The model under review builds one solid part; all positions refer to its coordinate system, in mm. Coordinates: 2 decimals unless noted, no trailing zeros. Loops run counter-clockwise (first coordinate to the right, second up) from the corner with the lowest first, then second, coordinate; pieces in that order, holes last. Notation, with made-up numbers: M -21.75,18 L 12.25,18 A15 cw 12.25,33 Z; hole C 52,16.5 d2. An arc over 180 degrees is marked long. Use CSV: the item, a comma, the result in double quotes. Start each with the question number.
from build123d import *

# Parameters (mm, degrees)
SKETCH_1_R          = 6
EXTRUDE_1_DEPTH     = 3
SKETCH_2_R          = 2.5
SKETCH_2_W          = 12
SKETCH_2_H          = 28
SKETCH_2_W_2        = 10
CUT_EXTRUDE_1_DEPTH = 725.098439741
SKETCH_3_W          = 6.5
SKETCH_3_H          = 275.47
EXTRUDE_2_DEPTH     = 3
SKETCH_4_W          = 602.3
SKETCH_4_H          = 15
EXTRUDE_3_DEPTH     = 3
FILLET_1_R          = 4


with BuildPart() as part:
    # 草图1 → 凸台-拉伸1 (new body)
    with BuildSketch(Plane.XY):
        with BuildLine():
            Line((64.592959067, -287.27493325), (-37.121356584, -436.580350718))
            ThreePointArc((-37.121356584, -436.580350718), (-39.401099826, -438.618784839), (-42.369287668, -439.355197667))
            Line((-42.369287668, -439.355197667), (-87.565404468, -439.355197667))
            ThreePointArc((-87.565404468, -439.355197667), (-90.533592309, -438.618784839), (-92.813335552, -436.580350718))
            Line((-92.813335552, -436.580350718), (-194.527651202, -287.27493325))
            Line((-194.527651202, -287.27493325), (-376.117346068, -287.27493325))
            Line((-376.117346068, -287.27493325), (-376.117346068, -612.39493325))
            ThreePointArc((-376.117346068, -612.39493325), (-374.257474128, -616.885061311), (-369.767346068, -618.74493325))
            Line((-369.767346068, -618.74493325), (239.832653932, -618.74493325))
            ThreePointArc((239.832653932, -618.74493325), (244.322781993, -616.885061311), (246.182653932, -612.39493325))
            Line((246.182653932, -612.39493325), (246.182653932, -287.27493325))
            Line((246.182653932, -287.27493325), (64.592959067, -287.27493325))
        make_face()
        with Locations((-111.371152168, -477.768197584)):
            Circle(SKETCH_1_R, mode=Mode.SUBTRACT)
        with Locations((-18.563539968, -477.768197584)):
            Circle(SKETCH_1_R, mode=Mode.SUBTRACT)
        with Locations((239.832653932, -607.63243325)):
            Circle(SKETCH_1_R, mode=Mode.SUBTRACT)
        with Locations((239.832653932, -594.93243325)):
            Circle(SKETCH_1_R, mode=Mode.SUBTRACT)
        with Locations(Location((-369.767346068, -607.63243325, 0), (0, 0, 180))):
            Circle(SKETCH_1_R, mode=Mode.SUBTRACT)
        with Locations(Location((-369.767346068, -594.93243325, 0), (0, 0, 180))):
            Circle(SKETCH_1_R, mode=Mode.SUBTRACT)
        with BuildLine():
            Line((-120.598278576, -553.999595792), (-117.888346515, -540.449935487))
            Line((-117.888346515, -540.449935487), (-113.593422095, -518.975313388))
            Line((-113.593422095, -518.975313388), (-109.909811627, -500.557261048))
            ThreePointArc((-109.909811627, -500.557261048), (-109.015545442, -498.354731753), (-107.373986867, -496.635390964))
            Line((-107.373986867, -496.635390964), (-68.658208598, -468.981263629))
            ThreePointArc((-68.658208598, -468.981263629), (-64.967346068, -467.798471171), (-61.276483538, -468.981263629))
            Line((-61.276483538, -468.981263629), (-22.560705269, -496.635390964))
            ThreePointArc((-22.560705269, -496.635390964), (-20.919146693, -498.354731753), (-20.024880508, -500.557261048))
            Line((-20.024880508, -500.557261048), (-16.34127004, -518.975313388))
            Line((-16.34127004, -518.975313388), (-12.04634562, -540.449935487))
            Line((-12.04634562, -540.449935487), (-9.336413559, -553.999595792))
            ThreePointArc((-9.336413559, -553.999595792), (-10.652378252, -559.270762801), (-15.56310085, -561.59493325))
            Line((-15.56310085, -561.59493325), (-114.371591285, -561.59493325))
            ThreePointArc((-114.371591285, -561.59493325), (-119.282313883, -559.270762801), (-120.598278576, -553.999595792))
        make_face(mode=Mode.SUBTRACT)
    extrude(amount=EXTRUDE_1_DEPTH)

    # 草图2 → 切除-拉伸1 (cut, through all)
    with BuildSketch(Plane.XY.offset(3)):
        with Locations((-193.155157013, -305.27493325)):
            Circle(SKETCH_2_R)
        with Locations((-108.702722738, -429.24180925)):
            Circle(SKETCH_2_R)
        with Locations((-150.928939875, -367.25837125)):
            Circle(SKETCH_2_R)
        with Locations((-326.117346068, -609.74493325)):
            Circle(SKETCH_2_R)
        with Locations((-367.117346068, -338.74493325)):
            Circle(SKETCH_2_R)
        with Locations((-367.117346068, -538.74493325)):
            Circle(SKETCH_2_R)
        with Locations((-367.117346068, -438.74493325)):
            Circle(SKETCH_2_R)
        with Locations((-126.117346068, -609.74493325)):
            Circle(SKETCH_2_R)
        with Locations((-226.117346068, -609.74493325)):
            Circle(SKETCH_2_R)
        with Locations(Location((-21.231969397, -429.24180925, 0), (0, 0, 180))):
            Circle(SKETCH_2_R)
        with Locations(Location((20.99424774, -367.25837125, 0), (0, 0, 180))):
            Circle(SKETCH_2_R)
        with Locations(Location((63.220464877, -305.27493325, 0), (0, 0, 180))):
            Circle(SKETCH_2_R)
        with Locations(Location((237.182653932, -338.74493325, 0), (0, 0, 180))):
            Circle(SKETCH_2_R)
        with Locations(Location((237.182653932, -438.74493325, 0), (0, 0, 180))):
            Circle(SKETCH_2_R)
        with Locations(Location((237.182653932, -538.74493325, 0), (0, 0, 180))):
            Circle(SKETCH_2_R)
        with Locations(Location((196.182653932, -609.74493325, 0), (0, 0, 180))):
            Circle(SKETCH_2_R)
        with Locations(Location((96.182653932, -609.74493325, 0), (0, 0, 180))):
            Circle(SKETCH_2_R)
        with Locations(Location((-3.817346068, -609.74493325, 0), (0, 0, 180))):
            Circle(SKETCH_2_R)
        with Locations((240.182653932, -301.27493325)):
            Rectangle(SKETCH_2_W, SKETCH_2_H)
        with Locations((-370.117346068, -301.27493325)):
            Rectangle(SKETCH_2_W, SKETCH_2_H)
        with Locations((-371.117346068, -604.74493325)):
            Rectangle(SKETCH_2_W_2, SKETCH_2_H)
        with Locations((241.182653932, -604.74493325)):
            Rectangle(SKETCH_2_W_2, SKETCH_2_H)
    extrude(amount=-CUT_EXTRUDE_1_DEPTH, mode=Mode.SUBTRACT)

    # 草图3 → 凸台-拉伸2 (add)
    with BuildSketch(Plane.XY.offset(3)):
        Polygon((-109.909811627, -500.557261048), (-20.024880508, -500.557261048), (-20.024880508, -490.663105306), (-58.077135265, -460.679906373), (-109.015545442, -490.663105306), align=None)
        with Locations((-379.367346068, -453.00993325)):
            Rectangle(SKETCH_3_W, SKETCH_3_H)
        with Locations((249.432653932, -453.00993325)):
            Rectangle(SKETCH_3_W, SKETCH_3_H)
    extrude(amount=-EXTRUDE_2_DEPTH)

    # 草图4 → 凸台-拉伸3 (add)
    with BuildSketch(Plane.XY.offset(3)):
        with Locations((-64.967346068, -626.24493325)):
            Rectangle(SKETCH_4_W, SKETCH_4_H)
    extrude(amount=-EXTRUDE_3_DEPTH)

    # 圆角1
    fillet_1_edges = [part.edges().sort_by_distance(p)[0] for p in [
        (234.182653932, -287.27493325, 1.5),
        (-364.117346068, -287.27493325, 1.5),
        (252.682653932, -315.27493325, 1.5),
        (252.682653932, -590.74493325, 1.5),
        (-382.617346068, -590.74493325, 1.5),
        (-382.617346068, -315.27493325, 1.5),
        (-366.117346068, -633.74493325, 1.5),
        (236.182653932, -633.74493325, 1.5),
        (-20.024880508, -500.557261048, 1.5),
        (-109.909811627, -500.557261048, 1.5),
    ]]
    fillet(fillet_1_edges, radius=FILLET_1_R)


solid = part.part
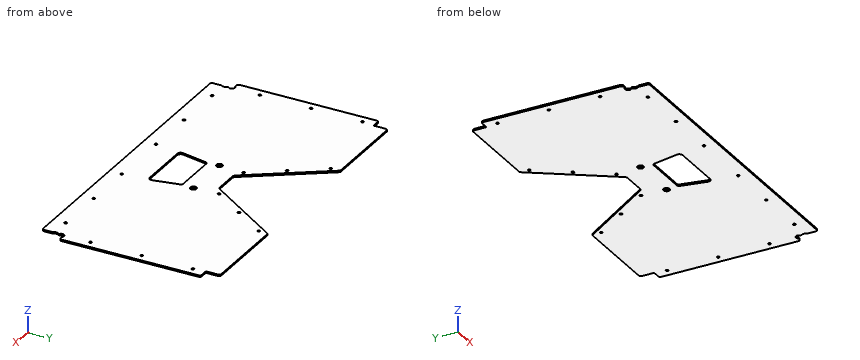
1. Add section A-A (x = -51.5). Write out the cut boundary in (y, z), plus the area to 3 significant figures.
2. Add section B-B (y = -400.5). Write out the cut boundary in (x, z), plus the area to 3 significant figures.
3. Add section C-C (z = 1.1). Give the number of separate pieces and of enclosed holes in the cut face, plus the area to 3 significant figures.
4. Insertion check: pin 1 Ø1.5 at (x, z) = (246, 1) entering from -Y. The pin has a flat end and moves straight along its axis. Give the tip position at first contact, or say it passes through.
5. To check wall thickness, follow line 1 along X through (y, z) = (-406, 1.9); line 2 along Y through (x, z) = (-107.5, 0.45); line 3 along X through (y, z) = (-441, 1.55). State the ranges of each line that lie inside material, in increasing order.
6. Add section D-D (x = 51.5). Write out the cut boundary in (y, z), plus the area to 3 significant figures.
Solved:
1,outline,"M -633.74,0 L -561.59,0 L -561.59,3 L -633.74,3 Z; M -500.56,0 L -439.36,0 L -439.36,3 L -500.56,3 Z"
1,area,"400 mm^2"
2,outline,"M -382.62,0 L -117.39,0 L -117.39,3 L -382.62,3 Z; M -12.54,0 L 252.68,0 L 252.68,3 L -12.54,3 Z"
2,area,"1,590 mm^2"
3,separate pieces,"1"
3,enclosed holes,"21"
3,area,"187,000 mm^2"
4,pin 1,"stops at y = -590.74"
5,line 1,"x = -382.62 to -113.65, -16.29 to 252.68"
5,line 2,"y = -633.74 to -561.59, -500.65 to -482.35, -473.18 to -431.43, -427.05 to -415.02"
5,line 3,"x = -382.62 to -368.2, -366.04 to 236.1, 238.26 to 252.68"
6,outline,"M -633.74,0 L -306.49,0 L -306.49,3 L -633.74,3 Z"
6,area,"982 mm^2"
